Could you check a few things on this model? Use its own coordinates, in mm. A direction names the side the tool comes from. Coordinates: 2 decimals unless noted, no trailing zeros. Write each loop counter-clockwise with the first axis right and the second up, starting at its lowest first coordinate (ties: lowest second). Pieces come first, ordered by that corner, then holes. Notation, with made-up numbers: (7.5, 25) - (59.5, 25) arc R14 ccw to (59.5, 32) - close; hole circle Ø11 at (-33, 61). An arc over 180 degrees is marked (long way). Answer as a JSON object with one key per item and string values. Group by question number.
1) Will these pins go through, and if not, where does the flat tip stop? pin 1 Ø3 at (x, z) = (5.5, 7) entering from +Y; pin 2 Ø4 at (x, y) = (0, 5.25) entering from +Z; pin 3 Ø1 at (y, z) = (-3.5, 3) entering from +X; pin 4 Ø2 at (y, z) = (-5, 3) entering from +X.
2) If we section it at A-A (x = 0): Write out the boundary of the cut face in (y, z), plus the area to 3 significant figures.
3) On a 3-axis mill with a long thin cutter (end or side, diameter ignored), from which of +Z, -Z, +X, -X, +Y, -Y can I reach the whole of each face in a straight line? I mean faces 1 (the flat face through (-1, 1, 9)), 2 (the flat face through (2, -8, 3)), 3 (the cylindrical face through (-1.72, -7.76, 7.48)). Say none if no direction works.
4) If we section it at C-C (z = 8): Write out the boundary of the cut face in (x, y), plus the area to 3 significant figures.
5) We'd pull the mould along X, two halves only. Please class faces 4 (the flat face through (2, -8, 6)), 5 (the cylindrical face through (-3.73, -1.74, 1.01)), 6 (the cylindrical face through (-1.72, -7.76, 1.48)): released by +X, released by -X, zero draft, split by the parting line, or undercut.
6) If we section it at D-D (y = -5): Write out the boundary of the cut face in (x, z).
7) Please list where these lines run through material, in increasing order: line 1 along Y through (x, z) = (0, 6.5); line 2 along Y through (x, z) = (0, 4.75); line 3 along Y through (x, z) = (3.5, 1.5).
8) If we section it at B-B (y = 5.25): Write out the boundary of the cut face in (x, z), plus the area to 3 significant figures.
```python
from build123d import *

# Parameters (mm, degrees)
F0_R      = 7.95
F1_DEPTH  = 3
F2_R      = 8.75
F2_R_2    = 7.95
F3_DEPTH  = 3
F4_R      = 7.95
F5_DEPTH  = 3
F6_R      = 1.5
F7_DEPTH  = 25
F8_R      = 7
F8_R_2    = 1.5
F8_R_3    = 3
F9_DEPTH  = 7
F10_R     = 1
F11_DEPTH = 25


with BuildPart() as f1:
    # F0 (on Top) → F1 (new body)
    with BuildSketch(Plane.XY):
        Circle(F0_R)
    extrude(amount=F1_DEPTH)

    # F2 (on face) → F3 (join)
    with BuildSketch(Plane.XY.offset(3)):
        Circle(F2_R)
        Circle(F2_R_2, mode=Mode.SUBTRACT)
        Circle(F2_R_2)
    extrude(amount=F3_DEPTH)

    # F4 (on face) → F5 (join)
    with BuildSketch(Plane.XY.offset(6)):
        Circle(F4_R)
    extrude(amount=F5_DEPTH)

    # F6 (on face) → F7 (cut)
    with BuildSketch(Plane.XY.offset(9)):
        with Locations((-4.104615283, 3.2733214598)):
            Circle(F6_R)
        with Locations((0, 5.25)):
            Circle(F6_R)
        with Locations((4.104615283, 3.2733214598)):
            Circle(F6_R)
        with Locations((5.118371539, -1.1682349033)):
            Circle(F6_R)
        with Locations((2.2778896304, -4.7300865565)):
            Circle(F6_R)
        with Locations((-2.2778896304, -4.7300865565)):
            Circle(F6_R)
        with Locations((-5.118371539, -1.1682349033)):
            Circle(F6_R)
    extrude(amount=-F7_DEPTH, mode=Mode.SUBTRACT)

    # F8 (on face) → F9 (cut)
    with BuildSketch(Plane.XY.offset(9)):
        Circle(F8_R)
        with Locations((-2.2778896304, -4.7300865565)):
            Circle(F8_R_2, mode=Mode.SUBTRACT)
        with Locations((-5.118371539, -1.1682349033)):
            Circle(F8_R_2, mode=Mode.SUBTRACT)
        with Locations((2.2778896304, -4.7300865565)):
            Circle(F8_R_2, mode=Mode.SUBTRACT)
        with Locations((5.118371539, -1.1682349033)):
            Circle(F8_R_2, mode=Mode.SUBTRACT)
        with Locations((-4.104615283, 3.2733214598)):
            Circle(F8_R_2, mode=Mode.SUBTRACT)
        Circle(F8_R_3, mode=Mode.SUBTRACT)
        with Locations((4.104615283, 3.2733214598)):
            Circle(F8_R_2, mode=Mode.SUBTRACT)
        with Locations((0, 5.25)):
            Circle(F8_R_2, mode=Mode.SUBTRACT)
    extrude(amount=-F9_DEPTH, mode=Mode.SUBTRACT)

    # F10 (on face) → F11 (cut)
    with BuildSketch(Plane.XY.offset(9)):
        Circle(F10_R)
    extrude(amount=-F11_DEPTH, mode=Mode.SUBTRACT)


solid = f1.part
```
Here are the results:
{
 "1": {"pin 1": "stops at y = 7.57", "pin 2": "stops at z = 9", "pin 3": "stops at x = 8.22", "pin 4": "stops at x = 7.78"},
 "2": {"outline": "(-8.75, 3) - (-7.95, 3) - (-7.95, 0) - (-1, 0) - (-1, 9) - (-3, 9) - (-3, 2) - (-7, 2) - (-7, 9) - (-7.95, 9) - (-7.95, 6) - (-8.75, 6) - close; (1, 0) - (3.75, 0) - (3.75, 2) - (3, 2) - (3, 9) - (1, 9) - close; (6.75, 0) - (7.95, 0) - (7.95, 3) - (8.75, 3) - (8.75, 6) - (7.95, 6) - (7.95, 9) - (7, 9) - (7, 2) - (6.75, 2) - close", "area": "67.9 mm²"},
 "3": {"face 1": "+Z, +X, -X, +Y, -Y", "face 2": "-Z", "face 3": "+Z"},
 "4": {"outline": "circle Ø15.9 at (0, 0); circle Ø6 at (0, 0); hole circle Ø14 at (0, 0); hole circle Ø2 at (0, 0)", "area": "69.8 mm²"},
 "5": {"face 4": "zero draft", "face 5": "undercut", "face 6": "split by the parting line"},
 "6": {"outline": "(-7.18, 3) - (-6.18, 3) - (-6.18, 0) - (-3.75, 0) - (-3.75, 2) - (-4.9, 2) - (-4.9, 9) - (-6.18, 9) - (-6.18, 6) - (-7.18, 6) - close; (-0.8, 0) - (0.8, 0) - (0.8, 2) - (-0.8, 2) - close; (3.75, 0) - (6.18, 0) - (6.18, 3) - (7.18, 3) - (7.18, 6) - (6.18, 6) - (6.18, 9) - (4.9, 9) - (4.9, 2) - (3.75, 2) - close"},
 "7": {"line 1": "y = -7.95 to -7, -3 to -1, 1 to 3, 7 to 7.95", "line 2": "y = -8.75 to -7, -3 to -1, 1 to 3, 7 to 8.75", "line 3": "y = -7.14 to -5.6, -3.86 to 1.9, 4.65 to 7.14"},
 "8": {"outline": "(-7, 3) - (-5.97, 3) - (-5.97, 0) - (-1.5, 0) - (-1.5, 2) - (-4.63, 2) - (-4.63, 9) - (-5.97, 9) - (-5.97, 6) - (-7, 6) - close; (1.5, 0) - (5.97, 0) - (5.97, 3) - (7, 3) - (7, 6) - (5.97, 6) - (5.97, 9) - (4.63, 9) - (4.63, 2) - (1.5, 2) - close", "area": "42.8 mm²"}
}
